Geometry: final body of the model. Coordinates: model frame, mm. A direction names the side the tool comes from. Give positions to 0.01 mm unless a question says otherwise; leave off trailing zeros. Write each loop counter-clockwise with the first axis right and the second up, starting at its lowest first coordinate (ties: lowest second). Pieces come first, ordered by that corner, then holes. Notation, with made-up numbers: (54.5, 74.25) -> (111.5, 74.25) arc R18 ccw to (111.5, 88.25) -> close; hole circle Ø2 at (-29, 13.25). An arc over 180 degrees is marked (long way). Answer in a Markdown table with one row per item. Add a question column.
Item 1: First-contact query: P1, Ø1, axis at x = 13, y = 4, coming from the -Z side; P2, Ø1.3, axis at x = 6.5, z = 13, coming from the +Y side; P3, Ø1.3, axis at x = 6.5, z = 13, coming from the -Y side; P4, Ø2.5, axis at x = 6.55, z = 0, coming from the -Y side. Flat tips, straight axial feed; report the tip coordinate or a pass-through.
Item 2: Section query A-A on z = 0. Output: boundary loops of the cut face in (x, y).
Item 3: Section query C-C on y = 5. Output: boundary loops of the cut face in (x, z), plus the area to 3 significant figures.
Item 4: Draft query along X for faces 4 (the flat face through (6, 8, 0)), 5 (the flat face through (5.497, 7, 13)), 6 (the flat face through (7, 2, 0)). Return one class per face: +X half, -X half, draft (parallel to the pull), parting line (faces both ways), or undercut.
Item 5: Access query for faces 1 (the flat face through (6, 7, 14.332)), 2 (the flat face through (7.146, 7, 13)), 3 (the cylindrical face through (5.57, 0.99, 0.22)). Directions: +Z, -Z, +X, -X, +Y, -Y. A direction counts if a zero-diameter tool reaches every point of the face in a straight line with its end or side. Return the directions, or none.
Item 6: Section query B-B on y = 3.5. Output: boundary loops of the cut face in (x, z).
Item 7: Material intervals for probe 1 along X at (y, z) = (1.1, 0); probe 2 along X at (y, z) = (1.5, 0); probe 3 along X at (y, z) = (0.5, -2.5), sorted ascending. Write a range as from..to.
```python
from build123d import *

# Parameters (mm, degrees)
SKETCH11_R          = 12
BOSS_EXTRUDE3_DEPTH = 2
BOSS_EXTRUDE4_START = -0.5
SKETCH12_W          = 1.649249379
SKETCH12_H          = 3.276759918
BOSS_EXTRUDE4_DEPTH = 1
SKETCH14_R          = 1
CUT_EXTRUDE2_DEPTH  = 2


with BuildPart() as part:
    # Sketch1 → Revolve1 (revolve)
    with BuildSketch(Plane.XY):
        Polygon((0.388993331, -0.067795133), (-5.226777212, -4), (6.321198199, -4), (6.321198199, 6), (-5.678801801, 6), align=None)
    revolve(axis=Axis((6.321198199, 11.047707555, 0), (0, -1, 0)))


with BuildPart() as body_2:
    # Split2: the piece on the far side of the plane
    add(part.part)
    split(bisect_by=Plane.ZX, keep=Keep.BOTTOM)


with BuildPart() as part_1:
    add(part.part)

    # Split2
    split(bisect_by=Plane.ZX, keep=Keep.TOP)

    # Sketch11 → Boss-Extrude3 (add)
    with BuildSketch(Plane(origin=(0, 6, 0), x_dir=(1, 0, 0), z_dir=(0, 1, 0))):
        with Locations(Location((6.321198199, 0, 0), (0, 0, 180))):
            Circle(SKETCH11_R)
    extrude(amount=BOSS_EXTRUDE3_DEPTH)

    # Sketch12 → Boss-Extrude4 (add)
    with BuildSketch(Plane(origin=(0, 8, 0), x_dir=(1, 0, 0), z_dir=(0, 1, 0)).offset(BOSS_EXTRUDE4_START)):
        with Locations((6.321198199, -12.693940914)):
            Rectangle(SKETCH12_W, SKETCH12_H)
    extrude(amount=-BOSS_EXTRUDE4_DEPTH)

    # Sketch14 → Cut-Extrude2 (cut)
    with BuildSketch(Plane(origin=(0, 0, 0), x_dir=(-1, 0, 0), z_dir=(0, -1, 0))):
        with Locations(Location((-6.546676473, 0, 0), (0, 0, 90))):
            Circle(SKETCH14_R)
    extrude(amount=-CUT_EXTRUDE2_DEPTH, mode=Mode.SUBTRACT)


solid = part_1.part
```
Findings below:
| question | item | result |
|---|---|---|
| 1 | P1 | stops at z = -8.22 |
| 1 | P2 | stops at y = 7.5 |
| 1 | P3 | stops at y = 6.5 |
| 1 | P4 | stops at y = 0 |
| 2 | outline | (-5.68, 6) -> (0.32, 0) -> (5.55, 0) -> (5.55, 2) -> (7.55, 2) -> (7.55, 0) -> (12.32, 0) -> (18.32, 6) -> (18.32, 8) -> (-5.68, 8) -> close |
| 3 | outline | circle Ø22 at (6.32, 0) |
| 3 | area | 380 mm^2 |
| 4 | face 4 | draft |
| 4 | face 5 | -X half |
| 4 | face 6 | undercut |
| 5 | face 1 | +Z, +X, -X, +Y, -Y |
| 5 | face 2 | +Z, +X, +Y, -Y |
| 5 | face 3 | -Y |
| 6 | outline | circle Ø19 at (6.32, 0) |
| 7 | probe 1 | x = -0.78..5.55, 7.55..13.42 |
| 7 | probe 2 | x = -1.18..5.55, 7.55..13.82 |
| 7 | probe 3 | x = 0.32..12.32 |
